Here's how the part is built. I have some questions about the finished solid (model axes, mm). A direction names the side the tool comes from. Give positions to 0.01 mm unless a question says otherwise; leave off trailing zeros. Loops run counter-clockwise (first coordinate to the right, second up) from the corner with the lowest first, then second, coordinate; pieces in that order, holes last. Notation, with made-up numbers: (-17, -19.5) - (28, -19.5) arc R21 ccw to (28, 6.5) - close; hole circle Ø2 at (74, -40). An arc over 180 degrees is marked (long way). Use a Markdown table: item, result.
from build123d import *

# Parameters (mm, degrees)
F0_R     = 6
F1_DEPTH = 2.5
F2_SIZE  = 5
F3_SIZE  = 1


with BuildPart() as f1:
    # F0 (on Front) → F1 (new body, symmetric)
    with BuildSketch(Plane.XZ):
        with BuildLine():
            Line((5, 40), (5, 30))
            Line((5, 30), (1.25, 30))
            ThreePointArc((1.25, 30), (0.883883, 29.116117), (0, 28.75))
            Line((0, 28.75), (0, 0))
            Line((0, 0), (0, -28.75))
            ThreePointArc((0, -28.75), (0.883883, -29.116117), (1.25, -30))
            Line((1.25, -30), (5, -30))
            Line((5, -30), (5, -40))
            Line((5, -40), (1.25, -40))
            ThreePointArc((1.25, -40), (0.883883, -40.883883), (0, -41.25))
            Line((0, -41.25), (0, -45))
            Line((0, -45), (25.368266, -45))
            Line((25.368266, -45), (25.368266, -24.494897))
            ThreePointArc((25.368266, -24.494897), (26.495282, -21.33262), (29.368266, -19.595918))
            ThreePointArc((29.368266, -19.595918), (45.368266, 0), (29.368266, 19.595918))
            ThreePointArc((29.368266, 19.595918), (26.495282, 21.33262), (25.368266, 24.494897))
            Line((25.368266, 24.494897), (25.368266, 45))
            Line((25.368266, 45), (0, 45))
            Line((0, 45), (0, 41.25))
            ThreePointArc((0, 41.25), (0.883883, 40.883883), (1.25, 40))
            Line((1.25, 40), (5, 40))
        make_face()
        with Locations((35, 0)):
            Circle(F0_R, mode=Mode.SUBTRACT)
        with BuildLine():
            Line((5, -30), (1.25, -30))
            ThreePointArc((1.25, -30), (0.883883, -30.883883), (0, -31.25))
            Line((0, -31.25), (0, -38.75))
            ThreePointArc((0, -38.75), (0.883883, -39.116117), (1.25, -40))
            Line((1.25, -40), (5, -40))
            Line((5, -40), (5, -30))
        make_face()
        with BuildLine():
            ThreePointArc((0, -31.25), (-0.883883, -30.883883), (-1.25, -30))
            Line((-1.25, -30), (-5, -30))
            Line((-5, -30), (-5, -40))
            Line((-5, -40), (-1.25, -40))
            ThreePointArc((-1.25, -40), (-0.883883, -39.116117), (0, -38.75))
            Line((0, -38.75), (0, -31.25))
        make_face()
        with BuildLine():
            Line((1.25, 30), (5, 30))
            Line((5, 30), (5, 40))
            Line((5, 40), (1.25, 40))
            ThreePointArc((1.25, 40), (0.883883, 39.116117), (0, 38.75))
            Line((0, 38.75), (0, 31.25))
            ThreePointArc((0, 31.25), (0.883883, 30.883883), (1.25, 30))
        make_face()
        with BuildLine():
            ThreePointArc((-1.25, 30), (-0.883883, 30.883883), (0, 31.25))
            Line((0, 31.25), (0, 38.75))
            ThreePointArc((0, 38.75), (-0.883883, 39.116117), (-1.25, 40))
            Line((-1.25, 40), (-5, 40))
            Line((-5, 40), (-5, 30))
            Line((-5, 30), (-1.25, 30))
        make_face()
    extrude(amount=F1_DEPTH, both=True)

    # F2
    f2_edges = [f1.edges().sort_by_distance(p)[0] for p in [
        (25.368266, 0, 45),
        (25.368266, 0, -45),
    ]]
    chamfer(f2_edges, length=F2_SIZE)

    # F3
    f3_edges = [f1.edges().sort_by_distance(p)[0] for p in [
        (-5, 0, 40),
        (-5, 0, -30),
        (-5, 0, 30),
        (-5, 0, -40),
    ]]
    chamfer(f3_edges, length=F3_SIZE)


solid = f1.part
(1) Suppose I cut it at A-A on z = 0. Write out the boundary of the cut face in (x, y).
A:
| item | result |
|---|---|
| outline | (0, -2.5) - (29, -2.5) - (29, 2.5) - (0, 2.5) - close; (41, -2.5) - (45.37, -2.5) - (45.37, 2.5) - (41, 2.5) - close |
(2) Suppose I cut it at D-D on x = 28. Write out the boundary of the cut face in (y, z), plus the area to 3 significant figures.
A:
| item | result |
|---|---|
| outline | (-2.5, -20.09) - (2.5, -20.09) - (2.5, 20.09) - (-2.5, 20.09) - close |
| area | 201 mm2 |
(3) If I drill on line 1 (X direction, y = 1.45, z = 37); line 2 (Z direction, x = 1, y = 1.6); line 3 (Z direction, x = 37, y = 1.1), over which ranges is the centre line in solid material (lowest first)?
A:
| item | result |
|---|---|
| line 1 | -5 to 25.37 |
| line 2 | -45 to -40.75, -39.25 to -30.75, -29.25 to 29.25, 30.75 to 39.25, 40.75 to 45 |
| line 3 | -16.27 to -5.66, 5.66 to 16.27 |
(4) Suppose I cut it at C-C on z = -26.5. Write out the boundary of the cut face in (x, y), plus the area to 3 significant figures.
A:
| item | result |
|---|---|
| outline | (0, -2.5) - (25.37, -2.5) - (25.37, 2.5) - (0, 2.5) - close |
| area | 127 mm2 |
(5) We'd pull the mould along Z, two halves only. Please class faces 5 (the face through (30.24, 0.04, -3.65)), 6 (the face through (45.365, -0.035, -0.383)), 7 (the face through (0, 0, 43)): pulls with the +Z half, pulls with the -Z half, needs draft (parallel to the pull), parting line crosses it, or undercut.
A:
| item | result |
|---|---|
| face 5 | undercut |
| face 6 | parting line crosses it |
| face 7 | needs draft |
(6) Suppose I cut it at B-B on x = 37. Write out the boundary of the cut face in (y, z).
A:
| item | result |
|---|---|
| outline | (-2.5, -16.27) - (2.5, -16.27) - (2.5, -5.66) - (-2.5, -5.66) - close; (-2.5, 5.66) - (2.5, 5.66) - (2.5, 16.27) - (-2.5, 16.27) - close |
(7) Will these pins go through, and if not, where does the flat tip stop? pin 1 (14 mm diameter, centred on x = 35, z = 0, fed in from +Y); pin 2 (2 mm diameter, centred on x = -3, y = -0.5, fed in from -Z); pin 3 (3 mm diameter, centred on x = -3, y = 0, fed in from +Z); pin 4 (1.1 mm diameter, centred on y = -1, z = -42.5, fed in from -X).
A:
| item | result |
|---|---|
| pin 1 | y = 2.5 |
| pin 2 | z = -40 |
| pin 3 | z = 40 |
| pin 4 | x = 0 |
(8) On a 3-axis mill with a long thin cutter (end or side, diameter ignored), from which of +Z, -Z, +X, -X, +Y, -Y can I reach the whole of each face in a straight line? I mean faces 1 (the face through (-3, 0, 40)), 2 (the face through (25.368, 0, -32)), 3 (the face through (25.368, 0, 32)), 4 (the face through (-3, 0, -40)). Say none if no direction works.
A:
| item | result |
|---|---|
| face 1 | +Z, -X, +Y, -Y |
| face 2 | -Z, +X, +Y, -Y |
| face 3 | +Z, +X, +Y, -Y |
| face 4 | -Z, -X, +Y, -Y |
